Source: CAD feature listing. Evaluate the final solid. Frame: model axes, mm. A direction names the side the tool comes from. Round coordinates to 2 decimals unless told otherwise and drop trailing zeros. Write each loop counter-clockwise with the first axis right and the second up, starting at its lowest first coordinate (ties: lowest second). Pieces come first, ordered by that corner, then holes. Notation, with made-up numbers: M 0,-15.75 L 9,-15.75 A19 cw 9,13.25 Z; hole C 26.25,57 d11. An arc over 180 degrees is marked long. Use a Markdown table: item, result.
Autodesk Inventor part; units mm, degrees
ref_plane "YZ Plane" through (0, 0, 0) normal (1, 0, 0) x (0, 1, 0)
ref_plane "XZ Plane" through (0, 0, 0) normal (0, 1, 0) x (-1, 0, 0)
ref_plane "XY Plane" through (0, 0, 0) normal (0, 0, 1) x (1, 0, 0)
sketch "Sketch1" plane through (0, 0, 0) normal (0, 0, 1) x (1, 0, 0)
  line L0 (19.05, -44.45) -> (-19.05, -44.45)
  line L1 (-19.05, -44.45) -> (-19.05, 44.45)
  line L2 (-19.05, 44.45) -> (19.05, 44.45)
  line L3 (19.05, 44.45) -> (19.05, -44.45)
  line L4 (19.05, -44.45) -> (-19.05, 44.45) construction
  line L5 (-19.05, -44.45) -> (19.05, 44.45) construction
  point P0 (0, 0)
  dimension "d0" = 38.1
  dimension "d1" = 88.9
extrude "Extrusion1" add sketch "Sketch1" along normal blind 673.8874
sketch "Sketch2" plane through (0, 0, 673.8874) normal (0, 0, 1) x (1, 0, 0)
  line L0 (19.05, -44.45) -> (19.05, 44.45)
  line L1 (19.05, 44.45) -> (-19.05, 44.45)
  line L2 (19.05, 31.75) -> (3.175, 31.75)
  line L3 (3.175, 31.75) -> (3.175, 28.575)
  line L4 (3.175, 28.575) -> (19.05, 28.575)
  line L5 (19.05, 28.575) -> (19.05, 31.75)
  point P0 (0, 0)
  dimension "d4" = 12.7
  dimension "d5" = 3.175
  dimension "d6" = 15.875
extrude "Extrusion2" cut sketch "Sketch2" against normal blind 736.6
sketch "Sketch4" plane through (19.05, -44.45, 673.8874) normal (1, 0, 0) x (0, 0, -1)
  line L0 (0, 0) -> (0, 73.025)
  line L1 (673.8874, 0) -> (0, 0)
  line L2 (673.8874, 73.025) -> (673.8874, 0)
  line L3 (673.8874, 6.35) -> (0, 6.35)
  line L4 (152.4, 6.35) -> (0, 47.1855)
  line L5 (250.444, 6.35) -> (421.8705, 26.67)
  line L6 (421.8705, 26.67) -> (673.8874, 26.67)
  point P0 (673.8874, 44.45)
  dimension "d15" = 6.35
  dimension "d20" = 152.4
  dimension "d21" = 165
  dimension "d23" = 20.32
  dimension "d24" = 98.044
  dimension "d25" = 173.24
extrude "Extrusion3" cut sketch "Sketch4" against normal blind 152.4
sketch "Sketch5" plane through (-19.05, 44.45, 0) normal (0, 1, 0) x (1, 0, 0)
  line L0 (38.1, -673.8874) -> (15.875, -673.8874)
  line L1 (15.875, -673.8874) -> (15.875, -572.2874)
  line L2 (15.875, -572.2874) -> (38.1, -572.2874)
  line L3 (38.1, -572.2874) -> (38.1, -673.8874)
  point P0 (19.05, 0)
  dimension "d28" = 22.225
  dimension "d29" = 101.6
extrude "Extrusion4" cut sketch "Sketch5" against normal blind 15.875
sketch "Sketch6" plane through (-19.05, 44.45, 0) normal (0, 1, 0) x (1, 0, 0)
  line L0 (38.1, 0) -> (38.1, -572.2874)
  line L1 (0, 0) -> (38.1, 0)
  line L2 (38.1, -215.9) -> (0, -215.9)
  line L3 (0, -215.9) -> (0, -342.9)
  line L4 (0, -342.9) -> (38.1, -342.9)
  line L5 (38.1, -342.9) -> (38.1, -215.9)
  point P0 (19.05, 0)
  dimension "d32" = 127
  dimension "d33" = 215.9
  dimension "d36" = 38.1
extrude "Extrusion5" cut sketch "Sketch6" against normal blind 15.875
properties part number "FrontSkid"
Q1. Section D-D on z = 382.5. Return loops of the section in (x, y) (3 decimals).
Results are:
| item | result |
|---|---|
| outline | M -19.05,-33.247 L 19.05,-33.247 L 19.05,28.575 L 3.175,28.575 L 3.175,31.75 L 19.05,31.75 L 19.05,44.45 L -19.05,44.45 Z |
Q2. Section A-A on x = 9. Give the number of separate pieces and of enclosed holes in the cut face, plus the area to 3 significant figures.
Results are:
| item | result |
|---|---|
| separate pieces | 3 |
| enclosed holes | 0 |
| area | 40,600 mm^2 |
Q3. Section C-C on z = 58. Return loops of the section in (x, y) (3 decimals), plus the area to 3 significant figures.
Results are:
| item | result |
|---|---|
| outline | M -19.05,-17.78 L 19.05,-17.78 L 19.05,28.575 L 3.175,28.575 L 3.175,31.75 L 19.05,31.75 L 19.05,44.45 L -19.05,44.45 Z |
| area | 2,320 mm^2 |
Q4. Line query: L1, parallel to Y at x = 4.5, z = 432 (3 decimals); L2, parallel to Z at x = 3, y = 29; L3, parallel to Y at x = 5, z = 123 (3 decimals). Output: solid intervals per line, ascending.
Results are:
| item | result |
|---|---|
| L1 | -38.1 to 28.575, 31.75 to 44.45 |
| L2 | 0 to 215.9, 342.9 to 572.29 |
| L3 | -17.78 to 28.575, 31.75 to 44.45 |
Q5. Reachability of faces 1 (the flat face through (0, 37, 342.9)), 2 (the flat face through (-3.175, 37, 624)), 3 (the flat face through (0, -17.78, 128)) from +Z, -Z, +X, -X, +Y, -Y: full face, straight path, thin tool, end or side. Return the list, or none.
Results are:
| item | result |
|---|---|
| face 1 | +X, -X, +Y |
| face 2 | +Z, +X, +Y |
| face 3 | -Z, +X, -X, -Y |
Q6. First-contact query: pin 1 Ø19 at (x, z) = (-1, 307) entering from +Y (3 decimals); pin 2 Ø6 at (x, z) = (1.5, 334) entering from -Y; pin 3 Ø3.5 at (y, z) = (29.5, 74.5) entering from +X; pin 4 Ø8 at (x, y) = (5.5, 37) entering from +Z. Flat tips, straight axial feed; report the tip coordinate or a pass-through.
Results are:
| item | result |
|---|---|
| pin 1 | y = 28.575 |
| pin 2 | y = -27.85 |
| pin 3 | x = 19.05 |
| pin 4 | z = 572.29 |
Q7. Section B-B on y = 38. Return loops of the section in (x, z) (3 decimals), plus the area to 3 significant figures.
Results are:
| item | result |
|---|---|
| outline | M -19.05,0 L 19.05,0 L 19.05,215.9 L -19.05,215.9 Z; M -19.05,342.9 L 19.05,342.9 L 19.05,572.287 L -3.175,572.287 L -3.175,673.887 L -19.05,673.887 Z |
| area | 18,600 mm^2 |
